from build123d import *

# Parameters (mm, degrees)
RESSALTO_EXTRUS_O1_DEPTH = 0.5


with BuildPart() as part:
    # Esboço1 → Ressalto-extrusão1 (new, symmetric)
    with BuildSketch(Plane(origin=(0, 0, 0), x_dir=(1, 0, 0), z_dir=(0, 1, 0))):
        Polygon((51.76515993, 74.050984143), (36.51515993, 74.050984143), (36.51515993, 84.183084139), (-6.48484007, 84.183084139), (-49.48484007, 84.183084139), (-49.48484007, 74.050984143), (-64.73484007, 74.050984143), (-64.73484007, 8.933084139), (-64.73484007, -60.318382682), (-21.48484007, -60.318382682), (-21.48484007, -69.817649271), (-21.48484007, -89.316915861), (-6.48484007, -89.316915861), (8.51515993, -89.316915861), (8.51515993, -69.817649271), (8.51515993, -60.318382682), (51.76515993, -60.318382682), (51.76515993, 8.933084139), align=None)
    extrude(amount=RESSALTO_EXTRUS_O1_DEPTH, both=True)


solid = part.part
Verification items for the finished model (mm, model axes). Coordinates: 2 decimals unless noted, no trailing zeros. Write each loop counter-clockwise with the first axis right and the second up, starting at its lowest first coordinate (ties: lowest second). Pieces come first, ordered by that corner, then holes. Notation, with made-up numbers: (-22, 3) - (34, 3) arc R23 cw to (34, 30) - close; hole circle Ø2 at (65, 83). An arc over 180 degrees is marked (long way). Answer as a JSON object with one key per item and string values.
(1) Cross-section at B-B on x = -32. Record the cut outline in (y, z), plus the area to 3 significant figures.
Report:
{"outline": "(-0.5, -84.18) - (0.5, -84.18) - (0.5, 60.32) - (-0.5, 60.32) - close", "area": "145 mm^2"}
(2) Thickness scan on line 1 along Z through (x, y) = (-56, 0.15); line 2 along Z through (x, y) = (19.5, 0). Record the ranges inside material, lowest first.
Report:
{"line 1": "-74.05 to 60.32", "line 2": "-84.18 to 60.32"}
(3) Cross-section at A-A on y = -0.05. Record the cut outline in (x, z), plus the area to 3 significant figures.
Report:
{"outline": "(-64.73, -74.05) - (-49.48, -74.05) - (-49.48, -84.18) - (36.52, -84.18) - (36.52, -74.05) - (51.77, -74.05) - (51.77, 60.32) - (8.52, 60.32) - (8.52, 89.32) - (-21.48, 89.32) - (-21.48, 60.32) - (-64.73, 60.32) - close", "area": "17,400 mm^2"}
(4) Cross-section at C-C on z = 78. Record the cut outline in (x, y), plus the area to 3 significant figures.
Report:
{"outline": "(-21.48, -0.5) - (8.52, -0.5) - (8.52, 0.5) - (-21.48, 0.5) - close", "area": "30.0 mm^2"}
